CAD build for the part. Positions are in the model's coordinates, mm. Round coordinates to 2 decimals unless told otherwise and drop trailing zeros. Use one line per item in the form item = value.
from build123d import *

# Parameters (mm, degrees)
SKETCH1_W           = 54.61
SKETCH1_H           = 28.575
SKETCH1_R           = 3.175
BOSS_EXTRUDE1_DEPTH = 3.175
SKETCH2_R           = 1.8415
CUT_EXTRUDE1_DEPTH  = 31.980256717
SKETCH4_R           = 1.8415
CUT_EXTRUDE2_DEPTH  = 31.980256717
SKETCH5_R           = 1.8415
CUT_EXTRUDE3_DEPTH  = 31.980256717


with BuildPart() as part:
    # Sketch1 → Boss-Extrude1 (new body)
    with BuildSketch(Plane.XY):
        Rectangle(SKETCH1_W, SKETCH1_H)
        with Locations((-10.795, 7.9375)):
            Circle(SKETCH1_R, mode=Mode.SUBTRACT)
    extrude(amount=BOSS_EXTRUDE1_DEPTH)

    # Sketch2 → Cut-Extrude1 (cut, through all)
    with BuildSketch(Plane.XY.offset(3.175)):
        with Locations((-23.495, 10.4775)):
            Circle(SKETCH2_R)
        with Locations((-23.495, -10.4775)):
            Circle(SKETCH2_R)
        with Locations((23.495, -10.4775)):
            Circle(SKETCH2_R)
        with Locations((23.495, 10.4775)):
            Circle(SKETCH2_R)
    extrude(amount=-CUT_EXTRUDE1_DEPTH, mode=Mode.SUBTRACT)

    # Sketch4 → Cut-Extrude2 (cut, through all)
    with BuildSketch(Plane.XY.offset(3.175)):
        with Locations((13.6525, 9.525)):
            Circle(SKETCH4_R)
    extrude(amount=-CUT_EXTRUDE2_DEPTH, mode=Mode.SUBTRACT)

    # Sketch5 → Cut-Extrude3 (cut, through all)
    with BuildSketch(Plane.XY.offset(3.175)):
        with Locations((-14.9225, -9.525)):
            Circle(SKETCH5_R)
        with Locations((13.6525, -9.525)):
            Circle(SKETCH5_R)
    extrude(amount=-CUT_EXTRUDE3_DEPTH, mode=Mode.SUBTRACT)


solid = part.part
1. Probe line 1 along X through (y, z) = (9.25, 0.3) (3 decimals); line 2 along Y through (x, z) = (23, 0.25); line 3 along Y through (x, z) = (-22, 2.05). List the from-to ranges inside material, lowest first. Write a range as from..to.
Completed:
line_1 = -27.305..-24.868, -22.122..-13.686, -7.904..11.832, 15.473..22.122, 24.868..27.305
line_2 = -14.29..-12.25, -8.7..8.7, 12.25..14.29
line_3 = -14.29..-11.55, -9.4..9.4, 11.55..14.29
2. Pull direction X, two halves, no side cores. Call faces 1 (the face through (-27.305, 0, 2)), 2 (the face through (14.64, -7.97, 1.61)), 3 (the face through (0, -14.288, 2)): +X half, -X half, draft (parallel to the pull), parting line (faces both ways), or undercut.
Completed:
face_1 = -X half
face_2 = undercut
face_3 = draft
3. Cut at A-A on z = 1.5. State how many separate pieces and enclosed holes the cut face has, and give its area (3 significant figures).
Completed:
separate_pieces = 1
enclosed_holes = 8
area = 1,450 mm2
